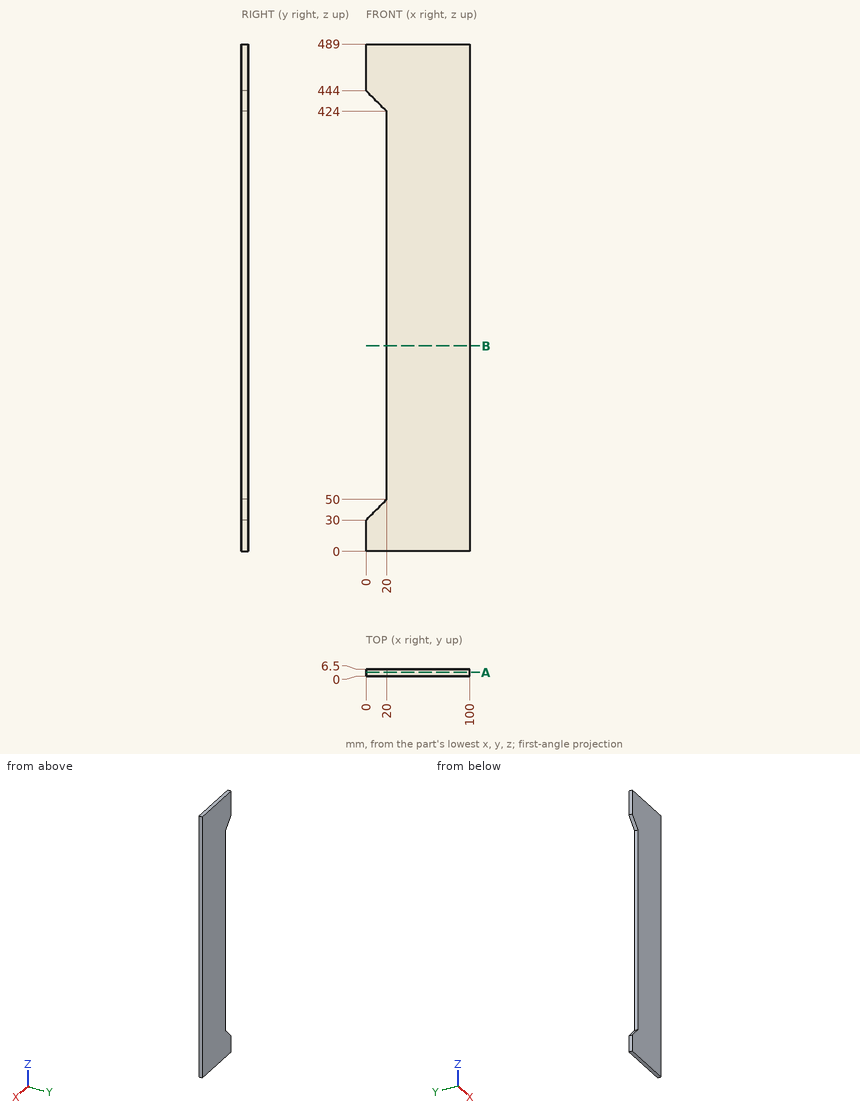
Input: dimensioned drawing with shaded views. Units: mm. Origin: part minimum x, y, z. Give positions to 0.01 mm unless a question says otherwise; leave off trailing zeros. Write each loop counter-clockwise with the first axis right and the second up, starting at its lowest first coordinate (ties: lowest second). Pieces come first, ordered by that corner, then holes.
1. Section query A-A, the plane y = 3.5. Return loops of the section in (x, z).
2. Line query: probe 1 along X at (y, z) = (3.75, 314); probe 2 along Z at (x, y) = (15.5, 0.75); probe 3 along X at (y, z) = (6.25, 34). Output: solid intervals per line, ascending.
3. Section query B-B, the plane z = 198. Return loops of the section in (x, y).
4. Pin query (flat end, axial travel): P1, Ø3, axis at y = 4.5, z = 391, coming from the -X side. Return the tip coordinate at first contact, or that it passes through.
Computed:
1. outline: (0, 0) - (100, 0) - (100, 489) - (0, 489) - (0, 444) - (20, 424) - (20, 50) - (0, 30) - close
2. probe 1: x = 20 to 100
2. probe 2: z = 0 to 45.5, 428.5 to 489
2. probe 3: x = 4 to 100
3. outline: (20, 0) - (100, 0) - (100, 6.5) - (20, 6.5) - close
4. P1: stops at x = 20
